CAD build for the part. Positions are in the model's coordinates, mm. A direction names the side the tool comes from. Coordinates: 2 decimals unless noted, no trailing zeros. Loops run counter-clockwise (first coordinate to the right, second up) from the corner with the lowest first, then second, coordinate; pieces in that order, holes last. Notation, with made-up numbers: (63.25, 40) -> (82.25, 40) arc R30 cw to (82.25, 70) -> close; hole circle Ø11 at (22, 40.5). An arc over 180 degrees is marked (long way). Write each question's results on one line, items separated by ' | '.
from build123d import *

# Parameters (mm, degrees)
SKETCH1_W                      = 12
SKETCH1_H                      = 10.5
BASE_DEPTH                     = 8.15
CONTACT_OPENING_DEPTH          = 9
CONTACT_OPENING_LEAD_IN_SIZE   = 0.5
SKETCH3_W                      = 5.6
SKETCH3_H                      = 3.18
CONTACT_AREA_DEPTH             = 8.5
CONTACT_AREA_LEAD_IN_SIZE      = 0.5
HOLDING_TINES_DEPTH            = 1.75
CONTACT_DEPTH                  = 0.375
CONTACT_PATTERN_COUNT          = 2
CONTACT_PATTERN_PITCH          = 2.5
TH_GROUND_LEGS_DEPTH           = 0.975
TH_GROUND_LEG_SHAPE_DEPTH      = 15.215776447
TH_GROUND_LEG_SHAPE_DEPTH_BACK = 15.215776447
TH_TAILS_DEPTH                 = 0.125
TH_TAILS_PATTERN_COUNT         = 2
TH_TAILS_PATTERN_PITCH         = 2


with BuildPart() as part:
    # Sketch1 → Base (new, symmetric)
    with BuildSketch(Plane.XY):
        Rectangle(SKETCH1_W, SKETCH1_H)
    extrude(amount=BASE_DEPTH, both=True)

    # Sketch2 → Contact Opening (cut)
    with BuildSketch(Plane.XY.offset(8.15)):
        with BuildLine():
            Line((-2.975, 4.33), (-4.225, 3.08))
            Line((-4.225, 3.08), (-4.225, -2.95))
            ThreePointArc((-4.225, -2.95), (-4.078553391, -3.303553391), (-3.725, -3.45))
            Line((-3.725, -3.45), (3.725, -3.45))
            ThreePointArc((3.725, -3.45), (4.078553391, -3.303553391), (4.225, -2.95))
            Line((4.225, -2.95), (4.225, 3.08))
            Line((4.225, 3.08), (2.975, 4.33))
            Line((2.975, 4.33), (-2.975, 4.33))
        make_face()
    extrude(amount=-CONTACT_OPENING_DEPTH, mode=Mode.SUBTRACT)

    # Contact Opening Lead-in
    contact_opening_lead_in_edges = [part.edges().sort_by_distance(p)[0] for p in [
        (0, 4.33, 8.15),
        (-3.6, 3.705, 8.15),
        (-4.225, 0.065, 8.15),
        (-4.078553391, -3.303553391, 8.15),
        (0, -3.45, 8.15),
        (4.078553391, -3.303553391, 8.15),
        (4.225, 0.065, 8.15),
        (3.6, 3.705, 8.15),
    ]]
    chamfer(contact_opening_lead_in_edges, length=CONTACT_OPENING_LEAD_IN_SIZE)

    # Sketch3 → Contact Area (add)
    with BuildSketch(Plane.XY.offset(-0.85)):
        with Locations((0, 0.44)):
            Rectangle(SKETCH3_W, SKETCH3_H)
    extrude(amount=CONTACT_AREA_DEPTH)

    # Contact Area Lead-in
    contact_area_lead_in_edges = [part.edges().sort_by_distance(p)[0] for p in [
        (-2.8, 0.44, 7.65),
        (0, -1.15, 7.65),
        (2.8, 0.44, 7.65),
        (0, 2.03, 7.65),
    ]]
    chamfer(contact_area_lead_in_edges, length=CONTACT_AREA_LEAD_IN_SIZE)

    # Sketch7 → Holding Tines (add, symmetric)
    with BuildSketch(Plane(origin=(0, 0, 0), x_dir=(1, 0, 0), z_dir=(0, 1, 0))):
        with BuildLine():
            Line((-4.225, -7.65), (-3.215243234, -4.951316752))
            ThreePointArc((-3.215243234, -4.951316752), (-3.027350135, -3.781276433), (-3.307189725, -2.629760924))
            Line((-3.307189725, -2.629760924), (-3.695, -1.8))
            Line((-3.695, -1.8), (-3.853538933, -1.874097279))
            Line((-3.853538933, -1.874097279), (-3.465728658, -2.703858203))
            ThreePointArc((-3.465728658, -2.703858203), (-3.202213044, -3.788201975), (-3.379145712, -4.889989942))
            Line((-3.379145712, -4.889989942), (-4.388902478, -7.588673189))
            Line((-4.388902478, -7.588673189), (-4.225, -7.65))
        make_face()
        with BuildLine():
            Line((4.225, -7.65), (4.388902478, -7.588673189))
            Line((4.388902478, -7.588673189), (3.379145712, -4.889989942))
            ThreePointArc((3.379145712, -4.889989942), (3.202213044, -3.788201975), (3.465728658, -2.703858203))
            Line((3.465728658, -2.703858203), (3.853538933, -1.874097279))
            Line((3.853538933, -1.874097279), (3.695, -1.8))
            Line((3.695, -1.8), (3.307189725, -2.629760924))
            ThreePointArc((3.307189725, -2.629760924), (3.027350135, -3.781276433), (3.215243234, -4.951316752))
            Line((3.215243234, -4.951316752), (4.225, -7.65))
        make_face()
    extrude(amount=HOLDING_TINES_DEPTH, both=True)

    # Sketch8 → Contact (add, symmetric)
    with BuildSketch(Plane(origin=(-1.25, 0, 0), x_dir=(0, 0, -1), z_dir=(1, 0, 0))):
        with BuildLine():
            Line((0.85, 2.03), (-2.595251124, 2.678262825))
            ThreePointArc((-2.595251124, 2.678262825), (-3.47053143, 2.712827451), (-4.318484282, 2.493086043))
            Line((-4.318484282, 2.493086043), (-5.65, 1.93))
            Line((-5.65, 1.93), (-5.581838417, 1.768819981))
            Line((-5.581838417, 1.768819981), (-4.250322699, 2.331906024))
            ThreePointArc((-4.250322699, 2.331906024), (-3.451833763, 2.538829183), (-2.627611475, 2.506280827))
            Line((-2.627611475, 2.506280827), (0.817639649, 1.858018002))
            Line((0.817639649, 1.858018002), (0.85, 2.03))
        make_face()
        with BuildLine():
            Line((-5.581838417, -0.888819981), (-5.65, -1.05))
            Line((-5.65, -1.05), (-4.318484282, -1.613086043))
            ThreePointArc((-4.318484282, -1.613086043), (-3.47053143, -1.832827451), (-2.595251124, -1.798262825))
            Line((-2.595251124, -1.798262825), (0.85, -1.15))
            Line((0.85, -1.15), (0.817639649, -0.978018002))
            Line((0.817639649, -0.978018002), (-2.627611475, -1.626280827))
            ThreePointArc((-2.627611475, -1.626280827), (-3.451833763, -1.658829183), (-4.250322699, -1.451906024))
            Line((-4.250322699, -1.451906024), (-5.581838417, -0.888819981))
        make_face()
    contact = extrude(amount=CONTACT_DEPTH, both=True)

    # Contact Pattern: Contact ×2
    with Locations(*[(i * CONTACT_PATTERN_PITCH, 0, 0) for i in range(1, CONTACT_PATTERN_COUNT)]):
        add(contact)

    # Sketch13 → TH Ground Legs (add, symmetric)
    with BuildSketch(Plane.XY.offset(-2.25)):
        with BuildLine():
            Line((6, -5.25), (6, -5.45))
            ThreePointArc((6, -5.45), (6.112536174, -5.84514538), (6.41637299, -6.121709028))
            Line((6.41637299, -6.121709028), (6.736045017, -6.280484954))
            ThreePointArc((6.736045017, -6.280484954), (7.400291967, -7.129098698), (7.157524757, -8.179066973))
            Line((7.157524757, -8.179066973), (6.527167526, -8.97))
            Line((6.527167526, -8.97), (6.23, -8.73316364))
            Line((6.23, -8.73316364), (6.860357231, -7.942230613))
            ThreePointArc((6.860357231, -7.942230613), (7.029323209, -7.211452694), (6.567007332, -6.620817528))
            Line((6.567007332, -6.620817528), (6.247335304, -6.462041602))
            ThreePointArc((6.247335304, -6.462041602), (5.789554503, -6.045352372), (5.62, -5.45))
            Line((5.62, -5.45), (5.62, -5.25))
            Line((5.62, -5.25), (6, -5.25))
        make_face()
        with BuildLine():
            Line((-5.62, -5.25), (-6, -5.25))
            Line((-6, -5.25), (-6, -5.45))
            ThreePointArc((-6, -5.45), (-6.112536174, -5.84514538), (-6.41637299, -6.121709028))
            Line((-6.41637299, -6.121709028), (-6.736045017, -6.280484954))
            ThreePointArc((-6.736045017, -6.280484954), (-7.400291967, -7.129098698), (-7.157524757, -8.179066973))
            Line((-7.157524757, -8.179066973), (-6.527167526, -8.97))
            Line((-6.527167526, -8.97), (-6.23, -8.73316364))
            Line((-6.23, -8.73316364), (-6.860357231, -7.942230613))
            ThreePointArc((-6.860357231, -7.942230613), (-7.029323209, -7.211452694), (-6.567007332, -6.620817528))
            Line((-6.567007332, -6.620817528), (-6.247335304, -6.462041602))
            ThreePointArc((-6.247335304, -6.462041602), (-5.789554503, -6.045352372), (-5.62, -5.45))
            Line((-5.62, -5.45), (-5.62, -5.25))
        make_face()
    extrude(amount=TH_GROUND_LEGS_DEPTH, both=True)

    # Sketch14 → TH Ground Leg Shape (cut, two sides: drawn at the far end of the back side and taken through both)
    with BuildSketch(Plane(origin=(0, 0, 0), x_dir=(0, 0, -1), z_dir=(1, 0, 0)).offset(-TH_GROUND_LEG_SHAPE_DEPTH_BACK)):
        with BuildLine():
            Line((3.225, -5.25), (3.225, -9))
            Line((3.225, -9), (1.275, -9))
            Line((1.275, -9), (1.275, -5.25))
            Line((1.275, -5.25), (1.755236252, -8.542172253))
            ThreePointArc((1.755236252, -8.542172253), (2.25, -8.97), (2.744763748, -8.542172253))
            Line((2.744763748, -8.542172253), (3.225, -5.25))
        make_face()
    extrude(amount=TH_GROUND_LEG_SHAPE_DEPTH + TH_GROUND_LEG_SHAPE_DEPTH_BACK, mode=Mode.SUBTRACT)

    # Sketch15 → TH Tails (add, symmetric)
    with BuildSketch(Plane(origin=(0, 0, -7.3), x_dir=(-1, 0, 0), z_dir=(0, 0, -1))):
        Polygon((-1.58, -5.25), (-0.92, -5.25), (-0.92, -8.1), (-1.041207868, -8.4), (-1.458792132, -8.4), (-1.58, -8.1), align=None)
        Polygon((0.92, -8.1), (1.041207868, -8.4), (1.458792132, -8.4), (1.58, -8.1), (1.58, -5.25), (0.92, -5.25), align=None)
    th_tails = extrude(amount=TH_TAILS_DEPTH, both=True)

    # TH Tails Pattern: TH Tails ×2
    with Locations(*[(0, 0, i * TH_TAILS_PATTERN_PITCH) for i in range(1, TH_TAILS_PATTERN_COUNT)]):
        add(th_tails)


solid = part.part
1) Two-plate mould, pull along Y, no slides. Class faces 1 (the cylindrical face through (-3.2, 0, 3.8)), 2 (the flat face through (0, 5.25, 0)), 3 (the flat face through (6, 0, 0)): pulls with the +Y half, pulls with the -Y half, needs draft (parallel to the pull), parting line crosses it, or undercut.
Outcome:
face 1: undercut | face 2: pulls with the +Y half | face 3: needs draft
2) Slice it at D-D (z = -6.5). Write the cut outline in (x, y).
Outcome:
outline: (-6, -5.25) -> (6, -5.25) -> (6, 5.25) -> (-6, 5.25) -> close
3) Pin check, flat tips, straight feed: pin 1 (4.5 mm diameter, centred on x = 1, z = 4, fed in from -Y); pin 2 (8 mm diameter, centred on y = -0.5, z = -1, fed in from +X); pin 3 (8 mm diameter, centred on y = 0, z = 2, fed in from -X). Stop position of each tip, or through.
Outcome:
pin 1: stops at y = -5.25 | pin 2: stops at x = 6 | pin 3: stops at x = -6
4) Drill centre lines: L1, parallel to X at y = -0.75, z = 0 (3 decimals); L2, parallel to Y at x = -0.25, z = 3.25; L3, parallel to Z at x = 1.5, y = -7.75 (3 decimals). Where is each one in solid material? Low to high. Write a range as from..to.
Outcome:
L1: x = -6..-4.225, -2.8..2.8, 4.225..6 | L2: y = -5.25..-3.45, -1.15..2.03, 4.33..5.25 | L3: z = -7.425..-7.175, -5.425..-5.175
5) Slice it at B-B (x = 0.5). Write the cut outline in (y, z).
Outcome:
outline: (-5.25, -8.15) -> (5.25, -8.15) -> (5.25, 8.15) -> (4.83, 8.15) -> (4.33, 7.65) -> (4.33, -0.85) -> (2.03, -0.85) -> (2.03, 7.15) -> (1.53, 7.65) -> (-0.65, 7.65) -> (-1.15, 7.15) -> (-1.15, -0.85) -> (-3.45, -0.85) -> (-3.45, 7.65) -> (-3.95, 8.15) -> (-5.25, 8.15) -> close
6) Slice it at A-A (z = 6.75). Write the cut outline in (x, y) (3 decimals), then the cut area to 3 significant figures.
Outcome:
outline: (-6, -5.25) -> (6, -5.25) -> (6, 5.25) -> (-6, 5.25) -> close; (-4.075, -1.75) -> (-3.888, -1.75) -> (-3.888, 1.75) -> (-4.075, 1.75) -> close; (-2.8, -1.15) -> (2.8, -1.15) -> (2.8, 2.03) -> (-2.8, 2.03) -> close; (3.888, -1.75) -> (4.075, -1.75) -> (4.075, 1.75) -> (3.888, 1.75) -> close; hole (-4.225, -2.95) arc R0.5 ccw to (-3.725, -3.45) -> (3.725, -3.45) arc R0.5 ccw to (4.225, -2.95) -> (4.225, 3.08) -> (2.975, 4.33) -> (-2.975, 4.33) -> (-4.225, 3.08) -> close | area: 81.0 mm^2
7) Which spindle directions (+Z, -Z, +X, -X, +Y, -Y) get a long thin tool onto all of the face, cutting with end or side? Do faces 4 (the conical face through (4.21, -3.44, 7.84)), 5 (the cylindrical face through (7.03, -7.22, -2.26)), 6 (the flat face through (0, -4.3, 8.15)), 7 (the flat face through (4.225, 0, 3)). Say none if no direction does.
Outcome:
face 4: +Z | face 5: +Z, -Z | face 6: +Z, +X, -X, +Y, -Y | face 7: none
